For this review, take the finished solid that the model builds, in its own axes (mm). A direction names the side the tool comes from. Round coordinates to 2 decimals unless told otherwise and drop trailing zeros. Order: outer loops, then holes, each group sorted by start corner. A loop starts at its lowest first (then second) coordinate and runs counter-clockwise, first axis right, second up. Notation, with made-up numbers: M 43,-22.5 L 75,-22.5 A24 cw 75,-1.5 Z; hole C 75.5,63.5 d2. An arc over 180 degrees is marked long. Answer as a JSON object with one key per item and string values.
from build123d import *

# Parameters (mm, degrees)
BOSS_EXTRUDE1_DEPTH = 1219.2
FILLET1_R           = 0.4064
SKETCH4_W           = 1898.4
SKETCH4_H           = 103.278519729
CUT_EXTRUDE1_DEPTH  = 60
SKETCH5_W           = 2.47699065
SKETCH5_H           = 2.94685794
CUT_EXTRUDE2_DEPTH  = 600
SKETCH8_R           = 1.65
CUT_EXTRUDE4_DEPTH  = 20
SKETCH9_R           = 1.65
CUT_EXTRUDE5_DEPTH  = 20
SKETCH10_R          = 1.65
CUT_EXTRUDE6_DEPTH  = 70
SKETCH11_R          = 1.65
CUT_EXTRUDE7_DEPTH  = 70


with BuildPart() as part:
    # Sketch3 → Boss-Extrude1 (new, symmetric)
    with BuildSketch(Plane.XY):
        Polygon((3.175, 25.4), (0, 25.4), (0, 0), (25.4, 0), (25.4, 3.175), (3.175, 3.175), align=None)
    extrude(amount=BOSS_EXTRUDE1_DEPTH, both=True)

    # Fillet1
    fillet1_edges = [part.edges().sort_by_distance(p)[0] for p in [
        (3.175, 3.175, 0),
    ]]
    fillet(fillet1_edges, radius=FILLET1_R)

    # Sketch4 → Cut-Extrude1 (cut)
    with BuildSketch(Plane.ZY):
        with Locations((-270, -26.239259864)):
            Rectangle(SKETCH4_W, SKETCH4_H)
    extrude(amount=-CUT_EXTRUDE1_DEPTH, mode=Mode.SUBTRACT)

    # Sketch5 → Cut-Extrude2 (cut)
    with BuildSketch(Plane(origin=(0, 0, 679.2), x_dir=(-1, 0, 0), z_dir=(0, 0, -1))):
        with Locations((-4.413495325, 4.64842897)):
            Rectangle(SKETCH5_W, SKETCH5_H)
    extrude(amount=-CUT_EXTRUDE2_DEPTH, mode=Mode.SUBTRACT)

    # Sketch8 → Cut-Extrude4 (cut)
    with BuildSketch(Plane(origin=(3.175, 0, 0), x_dir=(0, 0, -1), z_dir=(1, 0, 0))):
        with Locations(Location((-1179.2, 10.675, 0), (0, 0, 90))):
            Circle(SKETCH8_R)
        with Locations(Location((-1159.2, 10.675, 0), (0, 0, 90))):
            Circle(SKETCH8_R)
        with Locations(Location((-1139.2, 10.675, 0), (0, 0, 90))):
            Circle(SKETCH8_R)
        with Locations(Location((-1119.2, 10.675, 0), (0, 0, 90))):
            Circle(SKETCH8_R)
        with Locations(Location((-1099.2, 10.675, 0), (0, 0, 90))):
            Circle(SKETCH8_R)
        with Locations(Location((-1079.2, 10.675, 0), (0, 0, 90))):
            Circle(SKETCH8_R)
        with Locations(Location((-1059.2, 10.675, 0), (0, 0, 90))):
            Circle(SKETCH8_R)
        with Locations(Location((-1039.2, 10.675, 0), (0, 0, 90))):
            Circle(SKETCH8_R)
        with Locations(Location((-1019.2, 10.675, 0), (0, 0, 90))):
            Circle(SKETCH8_R)
        with Locations(Location((-999.2, 10.675, 0), (0, 0, 90))):
            Circle(SKETCH8_R)
        with Locations(Location((-979.2, 10.675, 0), (0, 0, 90))):
            Circle(SKETCH8_R)
        with Locations(Location((-959.2, 10.675, 0), (0, 0, 90))):
            Circle(SKETCH8_R)
        with Locations(Location((-939.2, 10.675, 0), (0, 0, 90))):
            Circle(SKETCH8_R)
        with Locations(Location((-919.2, 10.675, 0), (0, 0, 90))):
            Circle(SKETCH8_R)
        with Locations(Location((-899.2, 10.675, 0), (0, 0, 90))):
            Circle(SKETCH8_R)
        with Locations(Location((-879.2, 10.675, 0), (0, 0, 90))):
            Circle(SKETCH8_R)
        with Locations(Location((-859.2, 10.675, 0), (0, 0, 90))):
            Circle(SKETCH8_R)
        with Locations(Location((-839.2, 10.675, 0), (0, 0, 90))):
            Circle(SKETCH8_R)
        with Locations(Location((-819.2, 10.675, 0), (0, 0, 90))):
            Circle(SKETCH8_R)
        with Locations(Location((-799.2, 10.675, 0), (0, 0, 90))):
            Circle(SKETCH8_R)
        with Locations(Location((-779.2, 10.675, 0), (0, 0, 90))):
            Circle(SKETCH8_R)
        with Locations(Location((-759.2, 10.675, 0), (0, 0, 90))):
            Circle(SKETCH8_R)
        with Locations(Location((-739.2, 10.675, 0), (0, 0, 90))):
            Circle(SKETCH8_R)
        with Locations(Location((-719.2, 10.675, 0), (0, 0, 90))):
            Circle(SKETCH8_R)
    extrude(amount=-CUT_EXTRUDE4_DEPTH, mode=Mode.SUBTRACT)

    # Sketch9 → Cut-Extrude5 (cut)
    with BuildSketch(Plane(origin=(0, 3.175, 0), x_dir=(1, 0, 0), z_dir=(0, 1, 0))):
        with Locations(Location((10.675, -1179.2, 0), (0, 0, 180))):
            Circle(SKETCH9_R)
        with Locations(Location((10.675, -1159.2, 0), (0, 0, 180))):
            Circle(SKETCH9_R)
        with Locations(Location((10.675, -1139.2, 0), (0, 0, 180))):
            Circle(SKETCH9_R)
        with Locations(Location((10.675, -1119.2, 0), (0, 0, 180))):
            Circle(SKETCH9_R)
        with Locations(Location((10.675, -1099.2, 0), (0, 0, 180))):
            Circle(SKETCH9_R)
        with Locations(Location((10.675, -1079.2, 0), (0, 0, 180))):
            Circle(SKETCH9_R)
        with Locations(Location((10.675, -1059.2, 0), (0, 0, 180))):
            Circle(SKETCH9_R)
        with Locations(Location((10.675, -1039.2, 0), (0, 0, 180))):
            Circle(SKETCH9_R)
        with Locations(Location((10.675, -1019.2, 0), (0, 0, 180))):
            Circle(SKETCH9_R)
        with Locations(Location((10.675, -999.2, 0), (0, 0, 180))):
            Circle(SKETCH9_R)
        with Locations(Location((10.675, -979.2, 0), (0, 0, 180))):
            Circle(SKETCH9_R)
        with Locations(Location((10.675, -959.2, 0), (0, 0, 180))):
            Circle(SKETCH9_R)
        with Locations(Location((10.675, -939.2, 0), (0, 0, 180))):
            Circle(SKETCH9_R)
        with Locations(Location((10.675, -919.2, 0), (0, 0, 180))):
            Circle(SKETCH9_R)
        with Locations(Location((10.675, -899.2, 0), (0, 0, 180))):
            Circle(SKETCH9_R)
        with Locations(Location((10.675, -879.2, 0), (0, 0, 180))):
            Circle(SKETCH9_R)
        with Locations(Location((10.675, -859.2, 0), (0, 0, 180))):
            Circle(SKETCH9_R)
        with Locations(Location((10.675, -839.2, 0), (0, 0, 180))):
            Circle(SKETCH9_R)
        with Locations(Location((10.675, -819.2, 0), (0, 0, 180))):
            Circle(SKETCH9_R)
        with Locations(Location((10.675, -799.2, 0), (0, 0, 180))):
            Circle(SKETCH9_R)
        with Locations(Location((10.675, -779.2, 0), (0, 0, 180))):
            Circle(SKETCH9_R)
        with Locations(Location((10.675, -759.2, 0), (0, 0, 180))):
            Circle(SKETCH9_R)
        with Locations(Location((10.675, -739.2, 0), (0, 0, 180))):
            Circle(SKETCH9_R)
        with Locations(Location((10.675, -719.2, 0), (0, 0, 180))):
            Circle(SKETCH9_R)
    extrude(amount=-CUT_EXTRUDE5_DEPTH, mode=Mode.SUBTRACT)

    # Sketch10 → Cut-Extrude6 (cut)
    with BuildSketch(Plane(origin=(3.175, 0, 0), x_dir=(0, 0, -1), z_dir=(1, 0, 0))):
        with Locations(Location((-1200.15, 11.9634, 0), (0, 0, 90))):
            Circle(SKETCH10_R)
        with Locations(Location((-698.25, 11.9634, 0), (0, 0, 90))):
            Circle(SKETCH10_R)
    extrude(amount=-CUT_EXTRUDE6_DEPTH, mode=Mode.SUBTRACT)

    # Sketch11 → Cut-Extrude7 (cut)
    with BuildSketch(Plane(origin=(0, 3.175, 0), x_dir=(1, 0, 0), z_dir=(0, 1, 0))):
        with Locations(Location((10.364377143, -691.195704333, 0), (0, 0, 180))):
            Circle(SKETCH11_R)
        with Locations(Location((12.7, -1207.204295667, 0), (0, 0, 180))):
            Circle(SKETCH11_R)
    extrude(amount=-CUT_EXTRUDE7_DEPTH, mode=Mode.SUBTRACT)


solid = part.part
1) For L1, parallel to Z at x = 12.5, y = 2; L2, parallel to X at y = 0.9, z = 1039.2 (3 decimals); L3, parallel to Y at x = 12.5, z = 1148 (3 decimals), list the stretches that pass through material, from the lowest coordinate up.
Geometry check:
{"L1": "z = 679.2 to 1205.57, 1208.84 to 1219.2", "L2": "x = 0 to 9.025, 12.325 to 25.4", "L3": "y = 0 to 3.175"}
2) Add section A-A on z = 749.5. State the section outline as (x, y) points (3 decimals).
Geometry check:
{"outline": "M 0,0 L 25.4,0 L 25.4,3.175 L 3.175,3.175 L 3.175,25.4 L 0,25.4 Z"}
3) Machinability: for faces 1 (the flat face through (0, 13, 953)), 2 (the flat face through (3.175, 14, 953)), which of the approach directions +Z, -Z, +X, -X, +Y, -Y give a long, thin tool a straight path to every point of the face, cutting with its end or side? Answer none if there is none.
Geometry check:
{"face 1": "+Z, -Z, -X, +Y, -Y", "face 2": "+Z, -Z, +X, +Y"}
4) Insertion check: P1, Ø1, axis at x = 4, y = 12, coming from the +Z side; P2, Ø4, axis at y = 17.5, z = 807.5, coming from the +X side (3 decimals); P3, Ø5, axis at x = 9, z = 1012, coming from the +Y side (3 decimals). Each pin has a flat end and moves straight along its axis. Give the tip position at first contact, or say it passes through.
Geometry check:
{"P1": "passes through", "P2": "stops at x = 3.175", "P3": "stops at y = 3.175"}
